Here's how the part is built. I have some questions about the finished solid (model axes, mm). A direction names the side the tool comes from. Round coordinates to 2 decimals unless told otherwise and drop trailing zeros. Loops run counter-clockwise (first coordinate to the right, second up) from the corner with the lowest first, then second, coordinate; pieces in that order, holes last. Notation, with made-up numbers: M 78,25.25 L 124,25.25 A27 ccw 124,42.25 Z; hole C 74,33.5 d1. An arc over 180 degrees is marked long. One line per question, with ' | ' between items. Start each with the question number.
Autodesk Inventor part; units mm, degrees
ref_plane "YZ Plane" through (0, 0, 0) normal (1, 0, 0) x (0, 1, 0)
ref_plane "XZ Plane" through (0, 0, 0) normal (0, 1, 0) x (-1, 0, 0)
ref_plane "XY Plane" through (0, 0, 0) normal (0, 0, 1) x (1, 0, 0)
sketch "Boceto1" plane through (0, 0, 0) normal (0, 1, 0) x (-1, 0, 0)
  line L0 (0, 0) -> (80, 0)
  line L1 (80, 0) -> (80, -80)
  line L2 (80, -80) -> (0, -80)
  line L3 (0, -80) -> (0, 0)
  line L4 (10, -70) -> (70, -70)
  line L5 (70, -70) -> (70, -10)
  line L6 (70, -10) -> (10, -10)
  line L7 (10, -10) -> (10, -70)
  line L8 (0, -12.375) -> (80, -12.375)
  line L9 (0, -14.95) -> (80, -14.95)
  line L10 (0, -17.525) -> (80, -17.525)
  line L11 (80, -20.1) -> (0, -20.1)
  line L12 (0, -22.675) -> (80, -22.675)
  line L13 (0, -12.575) -> (80, -12.575)
  line L14 (0, -15.15) -> (80, -15.15)
  line L15 (0, -17.725) -> (80, -17.725)
  line L16 (80, -20.3) -> (0, -20.3)
  line L17 (0, -22.875) -> (80, -22.875)
  line L18 (0, -25.25) -> (80, -25.25)
  line L19 (0, -25.45) -> (80, -25.45)
  line L20 (10, -40) -> (80, -40)
  line L21 (0, -67.625) -> (80, -67.625)
  line L22 (0, -65.05) -> (80, -65.05)
  line L23 (0, -62.475) -> (80, -62.475)
  line L24 (80, -59.9) -> (0, -59.9)
  line L25 (0, -57.325) -> (80, -57.325)
  line L26 (0, -67.425) -> (80, -67.425)
  line L27 (0, -64.85) -> (80, -64.85)
  line L28 (0, -62.275) -> (80, -62.275)
  line L29 (80, -59.7) -> (0, -59.7)
  line L30 (0, -57.125) -> (80, -57.125)
  line L31 (0, -54.75) -> (80, -54.75)
  line L32 (0, -54.55) -> (80, -54.55)
  line L33 (72.625, -7.375) -> (7.375, -7.375)
  line L34 (7.375, -7.375) -> (7.375, -72.625)
  line L35 (7.375, -72.625) -> (72.625, -72.625)
  line L36 (72.625, -72.625) -> (72.625, -7.375)
  line L37 (7.375, 0) -> (0, 0)
  line L38 (7.375, -80) -> (0, -80)
  point P0 (10, -12.375)
  point P1 (70, -12.375)
  point P2 (10, -14.95)
  point P3 (70, -14.95)
  point P4 (10, -17.525)
  point P5 (70, -17.525)
  point P6 (70, -20.1)
  point P7 (10, -20.1)
  point P8 (10, -22.675)
  point P9 (70, -22.675)
  point P10 (10, -12.575)
  point P11 (70, -12.575)
  point P12 (10, -15.15)
  point P13 (70, -15.15)
  point P14 (10, -17.725)
  point P15 (70, -17.725)
  point P16 (70, -20.3)
  point P17 (10, -20.3)
  point P18 (10, -22.875)
  point P19 (70, -22.875)
  point P20 (10, -25.25)
  point P21 (70, -25.25)
  point P22 (10, -25.45)
  point P23 (70, -25.45)
  point P24 (10, -67.625)
  point P25 (70, -67.625)
  point P26 (10, -65.05)
  point P27 (70, -65.05)
  point P28 (10, -62.475)
  point P29 (70, -62.475)
  point P30 (70, -59.9)
  point P31 (10, -59.9)
  point P32 (10, -57.325)
  point P33 (70, -57.325)
  point P34 (10, -67.425)
  point P35 (70, -67.425)
  point P36 (10, -64.85)
  point P37 (70, -64.85)
  point P38 (10, -62.275)
  point P39 (70, -62.275)
  point P40 (70, -59.7)
  point P41 (10, -59.7)
  point P42 (10, -57.125)
  point P43 (70, -57.125)
  point P44 (10, -54.75)
  point P45 (70, -54.75)
  point P46 (10, -54.55)
  point P47 (70, -54.55)
  point P48 (72.625, -12.375)
  point P49 (7.375, -12.375)
  point P50 (72.625, -54.55)
  point P51 (72.625, -25.45)
  point P52 (70, -25.45)
  point P53 (70, -54.55)
  point P54 (7.375, -25.45)
  point P55 (7.375, -54.55)
  point P56 (10, -54.55)
  point P57 (10, -25.45)
  point P58 (10, -67.625)
  point P59 (7.375, -67.625)
  point P60 (72.625, -67.625)
  point P61 (70, -67.625)
  point P62 (7.375, -14.95)
  point P63 (72.625, -14.95)
  point P64 (72.625, -65.05)
  point P65 (70, -65.05)
  point P66 (10, -65.05)
  point P67 (7.375, -65.05)
  point P68 (70, -67.425)
  point P69 (10, -67.425)
  point P70 (10, -12.575)
  point P71 (70, -12.575)
  point P72 (72.625, -64.85)
  point P73 (7.375, -64.85)
  point P74 (7.375, -15.15)
  point P75 (70, -15.15)
  point P76 (7.375, -62.475)
  point P77 (10, -64.85)
  point P78 (10, -62.475)
  point P79 (72.625, -62.475)
  point P80 (70, -62.475)
  point P81 (70, -64.85)
  point P82 (7.375, -17.525)
  point P83 (10, -15.15)
  point P84 (72.625, -17.525)
  dimension "d0" = 80
  dimension "d1" = 80
  dimension "d2" = 60
  dimension "d3" = 60
  dimension "d4" = 10
  dimension "d5" = 10
  dimension "d6" = 2.375
  dimension "d7" = 0.2
  dimension "d8" = 2.375
  dimension "d9" = 0.2
  dimension "d10" = 0.2
  dimension "d11" = 0.2
  dimension "d12" = 0.2
  dimension "d13" = 2.375
  dimension "d14" = 2.375
  dimension "d15" = 2.375
  dimension "d16" = 2.375
  dimension "d17" = 0.2
  dimension "d35" = 5
extrude "Extrusión1" add sketch "Boceto1" along normal blind 5 contours L0 L1 L8 L36 L33 L34 L3 | L8 L34 L13 L3 | L13 L34 L9 L3 | L34 L33 L36 L8 L5 L6 L7 | L8 L7 L13 L34 | L1 L13 L36 L8 | L13 L7 L9 L34 | L8 L5 L13 L7 | L7 L6 L5 L8 | L1 L9 L36 L13 | L36 L13 L5 L8 | L14 L34 L10 L3 | L13 L5 L9 L7 | L36 L9 L5 L13 | L14 L7 L10 L34 | L1 L10 L36 L14 | L15 L34 L11 L3 | L14 L5 L10 L7 | L36 L10 L5 L14 | L15 L7 L11 L34 | L1 L11 L36 L15 | L16 L34 L12 L3 | L15 L5 L11 L7 | L36 L11 L5 L15 | L16 L7 L12 L34 | L1 L12 L36 L16 | L17 L34 L18 L3 | L16 L5 L12 L7 | L36 L12 L5 L16 | L17 L7 L18 L34 | L1 L18 L36 L17 | L19 L34 L32 L3 | L17 L5 L18 L7 | L36 L18 L5 L17 | L19 L7 L32 L34 | L1 L20 L36 L19 | L31 L34 L30 L3 | L19 L5 L20 L7 | L1 L32 L36 L20 | L36 L20 L5 L19 | L31 L7 L30 L34 | L7 L20 L5 L32 | L36 L32 L5 L20 | L25 L34 L29 L3 | L31 L5 L30 L7 | L1 L30 L36 L31 | L25 L7 L29 L34 | L31 L36 L30 L5 | L24 L34 L28 L3 | L25 L5 L29 L7 | L1 L29 L36 L25 | L24 L7 L28 L34 | L25 L36 L29 L5 | L23 L34 L27 L3 | L24 L5 L28 L7 | L1 L28 L36 L24 | L23 L7 L27 L34 | L24 L36 L28 L5 | L22 L34 L26 L3 | L23 L5 L27 L7 | L1 L27 L36 L23 | L26 L34 L21 L3 | L22 L7 L26 L34 | L23 L36 L27 L5 | L21 L34 L35 L36 L1 L2 L3 | L26 L7 L21 L34 | L22 L5 L26 L7 | L1 L26 L36 L22 | L21 L7 L4 L5 L36 L35 L34 | L26 L5 L21 L7 | L22 L36 L26 L5 | L1 L21 L36 L26 | L21 L5 L4 L7 | L26 L36 L21 L5
sketch "Boceto2" plane through (0, 0, 0) normal (0, -1, 0) x (1, 0, 0)
  line L0 (0, -80) -> (-80, -80)
  line L1 (-80, 0) -> (0, 0)
  line L2 (-80, -80) -> (-80, 0)
  line L3 (-80, 0) -> (0, 0)
  line L4 (-80, -65.05) -> (0, -65.05) construction
  line L5 (0, 0) -> (0, -80)
  line L6 (-80, -80) -> (0, -80)
extrude "Extrusión4" add sketch "Boceto2" along normal blind 3
extrude "Extrusión5" add sketch "Boceto1" along normal blind 10 contours L34 L33 L36 L8 L5 L6 L7 | L8 L7 L13 L34 | L13 L7 L9 L34 | L8 L5 L13 L7 | L7 L6 L5 L8 | L36 L13 L5 L8 | L9 L7 L14 L34 | L13 L5 L9 L7 | L36 L9 L5 L13 | L14 L7 L10 L34 | L9 L5 L14 L7 | L36 L14 L5 L9 | L36 L10 L5 L14 | L19 L7 L32 L34 | L36 L20 L5 L19 | L36 L32 L5 L20 | L23 L7 L27 L34 | L27 L7 L22 L34 | L22 L7 L26 L34 | L27 L5 L22 L7 | L23 L36 L27 L5 | L26 L7 L21 L34 | L22 L5 L26 L7 | L27 L36 L22 L5 | L21 L7 L4 L5 L36 L35 L34 | L26 L5 L21 L7 | L22 L36 L26 L5 | L21 L5 L4 L7 | L26 L36 L21 L5
sketch "Boceto3" plane through (0, 10, 0) normal (0, 1, 0) x (1, 0, 0)
  line L0 (-7.375, 25.45) -> (-7.375, 54.55)
  line L1 (-7.375, 40) -> (-86.5517, 40)
  line L2 (-5, 39.5) -> (-84.1767, 39.5)
  line L3 (-5, 40.5) -> (-84.1767, 40.5)
  line L4 (-10, 54.55) -> (-10, 25.45)
  line L5 (-5, 40.5) -> (-5, 39.5)
  line L6 (-84.1767, 40.5) -> (-84.1767, 39.5)
  point P0 (0, 0)
  point P1 (-10, 40)
  point P2 (-10, 39.5)
  point P3 (-10, 40.5)
  point P4 (-7.375, 39.5)
  point P5 (-7.375, 40.5)
  dimension "d31" = 0.5
  dimension "d32" = 0.5
extrude "Extrusión6" cut sketch "Boceto3" against normal blind 2 contours L2 L4 L1 L0 | L1 L4 L3 L0 | L2 L6 L1 L4 | L1 L6 L3 L4
equation "\"d8\" = d6"
equation "\"d9\" = d7"
equation "\"d10\" = d9"
equation "\"d11\" = d7"
equation "\"d12\" = d7"
equation "\"d13\" = d6"
equation "\"d14\" = d6"
equation "\"d15\" = d6"
equation "\"d16\" = d6"
equation "\"d17\" = d7"
properties part number "Cortador Ancho PDMS5"
1) I'm going to push flat-ended pins straight in: pin 1 Ø1.5 at (x, y) = (-50, 2.5) entering from +Z; pin 2 Ø1.2 at (x, z) = (-5, -63.5) entering from +Y; pin 3 Ø2.5 at (y, z) = (7.5, -39.5) entering from +X (3 decimals); pin 4 Ø2.5 at (x, y) = (-43, 6.5) entering from -Z (3 decimals). Where does each tip first touch, or does it pass through?
2) We'd pull the mould along Z, two halves only. Please class faces 6 (the face through (-40, 5, -64)), 7 (the face through (-40, 10, -69)), 8 (the face through (-41, 1, 0)): pulls with the +Z half, pulls with the -Z half, needs draft (parallel to the pull), parting line crosses it, or undercut.
3) Imagine slicing it at C-C (y = 1.5). State how many separate pieces and enclosed holes the cut face has, then the cut area to 3 significant figures.
4) Please list where these lines run through material, in increasing order: L1, parallel to X at y = 6.75, z = -35 (3 decimals); L2, parallel to Y at x = -56, z = -64; L3, parallel to X at y = 9, z = -70 (3 decimals). Write a range as from..to.
5) For faces 1 (the face through (-76, 5, -40)), 2 (the face through (-76, 2, -15.15)), 3 (the face through (-80, 1, -41)), 4 (the face through (-10, 7, -16)), 5 (the face through (-39, 3, -54.55)), which set-ups out of +Z, -Z, +X, -X, +Y, -Y let a thin tool reach every point of the face, with its end or its side?
6) Imagine slicing it at D-D (z = -46.5). Write out the boundary of the cut face in (x, y) (3 decimals).
7) Imagine slicing it at B-B (z = -13.5). Write out the boundary of the cut face in (x, y) (3 decimals).
8) Imagine slicing it at A-A (y = 7). Write out the boundary of the cut face in (x, z) (3 decimals), then the cut area to 3 significant figures.
Results are:
1) pin 1: z = 0 | pin 2: y = 5 | pin 3: x = -7.375 | pin 4: z = -72.625
2) face 6: undercut | face 7: needs draft | face 8: pulls with the +Z half
3) separate pieces: 9 | enclosed holes: 0 | area: 6,270 mm²
4) L1: -72.625..-70, -10..-7.375 | L2: -3..5 | L3: -72.625..-7.375
5) face 1: +Z, -Z, -X, +Y | face 2: -X, +Y | face 3: +Z, -Z, -X, +Y, -Y | face 4: +Y | face 5: +X, -X, +Y
6) outline: M -80,-3 L 0,-3 L 0,5 L -7.375,5 L -7.375,10 L -10,10 L -10,5 L -70,5 L -70,10 L -72.625,10 L -72.625,5 L -80,5 Z
7) outline: M -80,-3 L 0,-3 L 0,5 L -7.375,5 L -7.375,10 L -72.625,10 L -72.625,5 L -80,5 Z
8) outline: M -72.625,-72.625 L -7.375,-72.625 L -7.375,-62.475 L -10,-62.475 L -10,-64.85 L -70,-64.85 L -70,-62.475 L -72.625,-62.475 Z; M -72.625,-54.55 L -70,-54.55 L -70,-25.45 L -72.625,-25.45 Z; M -72.625,-17.525 L -70,-17.525 L -70,-15.15 L -10,-15.15 L -10,-17.525 L -7.375,-17.525 L -7.375,-7.375 L -72.625,-7.375 Z; M -10,-54.55 L -7.375,-54.55 L -7.375,-25.45 L -10,-25.45 Z | area: 1,190 mm²
